Can you work these out from the model? Positions are in its coordinate system, mm. A direction names the side the tool comes from. Coordinates: 2 decimals unless noted, no trailing zeros. Order: outer loops, then holes, each group sorted by start corner. A loop starts at its lowest first (then second) coordinate and runs counter-clockwise, first axis right, second up. Notation, with made-up numbers: (76, -14) -> (133, -14) arc R16 ccw to (133, 3) -> close; hole circle Ø1 at (64, 48). An arc over 180 degrees is marked (long way). Answer in a Markdown table with one row per item.
```python
from build123d import *

# Parameters (mm, degrees)
SKETCH_2_W          = 37
SKETCH_2_H          = 13
EXTRUDE_2_DEPTH     = 3
SKETCH_3_R          = 1.5
CUT_EXTRUDE_2_DEPTH = 3
SKETCH_4_W          = 37
SKETCH_4_H          = 4
EXTRUDE_3_DEPTH     = 15
FILLET_4_R          = 3
FILLET_5_R          = 3
SKETCH_5_R          = 1.5
CUT_EXTRUDE_3_DEPTH = 10
FILLET_6_R          = 3


with BuildPart() as part:
    # 草图2 → 凸台-拉伸2 (new body)
    with BuildSketch(Plane(origin=(0, 0, 0), x_dir=(1, 0, 0), z_dir=(0, 1, 0))):
        Rectangle(SKETCH_2_W, SKETCH_2_H)
    extrude(amount=EXTRUDE_2_DEPTH)

    # 草图3 → 切除-拉伸2 (cut)
    with BuildSketch(Plane.XZ):
        with Locations(Location((-14.5, 0, 0), (0, 0, 270))):
            Circle(SKETCH_3_R)
        with Locations(Location((14.5, 0, 0), (0, 0, 270))):
            Circle(SKETCH_3_R)
    extrude(amount=-CUT_EXTRUDE_2_DEPTH, mode=Mode.SUBTRACT)

    # 草图4 → 凸台-拉伸3 (add)
    with BuildSketch(Plane.XZ):
        with Locations((0, -8.5)):
            Rectangle(SKETCH_4_W, SKETCH_4_H)
    extrude(amount=-EXTRUDE_3_DEPTH)

    # 圆角4
    fillet_4_edges = [part.edges().sort_by_distance(p)[0] for p in [
        (18.5, 15, -8.5),
    ]]
    fillet(fillet_4_edges, radius=FILLET_4_R)

    # 圆角5
    fillet_5_edges = [part.edges().sort_by_distance(p)[0] for p in [
        (-18.5, 15, -8.5),
    ]]
    fillet(fillet_5_edges, radius=FILLET_5_R)

    # 草图5 → 切除-拉伸3 (cut)
    with BuildSketch(Plane.XY.offset(-6.5)):
        with Locations((10, 9.01536156)):
            Circle(SKETCH_5_R)
        with Locations(Location((-10, 9.01536156, 0), (0, 0, 180))):
            Circle(SKETCH_5_R)
    extrude(amount=-CUT_EXTRUDE_3_DEPTH, mode=Mode.SUBTRACT)

    # 圆角6
    fillet_6_edges = [part.edges().sort_by_distance(p)[0] for p in [
        (-18.5, 1.5, 6.5),
        (18.5, 1.5, 6.5),
    ]]
    fillet(fillet_6_edges, radius=FILLET_6_R)


solid = part.part
```
(1) Suppose I cut it at A-A (x = 10). Please give me the cut outline in (y, z), and give its area (3 significant figures).
Response values:
| item | result |
|---|---|
| outline | (0, -10.5) -> (7.52, -10.5) -> (7.52, -6.5) -> (3, -6.5) -> (3, 6.5) -> (0, 6.5) -> close; (10.52, -10.5) -> (15, -10.5) -> (15, -6.5) -> (10.52, -6.5) -> close |
| area | 87.0 mm2 |
(2) I need wall thicknesses on line 1 (X direction, y = 1, z = 0); line 2 (Z direction, x = 8, y = 12.75); line 3 (Y direction, x = -5.5, z = 5.75). Which ranges of each line are inside material? Lowest first, please. Write a range as [from, to].
Response values:
| item | result |
|---|---|
| line 1 | [-18.5, -16], [-13, 13], [16, 18.5] |
| line 2 | [-10.5, -6.5] |
| line 3 | [0, 3] |
(3) We'd pull the mould along Z, two halves only. Please class faces 1 (the flat face through (0, 9, -6.5)), 2 (the cylindrical face through (17.64, 14.1, -8.47)), 3 (the cylindrical face through (-14.05, 1.48, -1.43)): +Z half, -Z half, draft (parallel to the pull), parting line (faces both ways), or undercut.
Response values:
| item | result |
|---|---|
| face 1 | +Z half |
| face 2 | draft |
| face 3 | undercut |
(4) Suppose I cut it at D-D (x = -14.5). Please give me the cut outline in (y, z), and give its area (3 significant figures).
Response values:
| item | result |
|---|---|
| outline | (0, -10.5) -> (15, -10.5) -> (15, -6.5) -> (3, -6.5) -> (3, -1.5) -> (0, -1.5) -> close; (0, 1.5) -> (3, 1.5) -> (3, 6.5) -> (0, 6.5) -> close |
| area | 90.0 mm2 |
(5) Suppose I cut it at B-B (y = 2.25). Please give me the cut outline in (x, z), and give its area (3 significant figures).
Response values:
| item | result |
|---|---|
| outline | (-18.5, -10.5) -> (18.5, -10.5) -> (18.5, 3.5) arc R3 ccw to (15.5, 6.5) -> (-15.5, 6.5) arc R3 ccw to (-18.5, 3.5) -> close; hole circle Ø3 at (-14.5, 0); hole circle Ø3 at (14.5, 0) |
| area | 611 mm2 |
(6) On a 3-axis mill with a long thin cutter (end or side, diameter ignored), from which of +Z, -Z, +X, -X, +Y, -Y can I reach the whole of each face in a straight line? I mean faces 4 (the flat face through (-18.5, 5, -7)), 5 (the flat face through (0, 3, 0)). Say none if no direction works.
Response values:
| item | result |
|---|---|
| face 4 | +Z, -Z, -X, +Y, -Y |
| face 5 | +Z, +X, -X, +Y |
(7) Suppose I cut it at C-C (z = 0). Please give me the cut outline in (x, y).
Response values:
| item | result |
|---|---|
| outline | (-18.5, 0) -> (-16, 0) -> (-16, 3) -> (-18.5, 3) -> close; (-13, 0) -> (13, 0) -> (13, 3) -> (-13, 3) -> close; (16, 0) -> (18.5, 0) -> (18.5, 3) -> (16, 3) -> close |
(8) Will these pins go through, and if not, where does the flat tip stop? pin 1 Ø2.5 at (x, z) = (-14.5, 0) entering from +Y; pin 2 Ø4 at (x, y) = (-12, 9) entering from +Z; pin 3 Ø1 at (x, z) = (2, -2) entering from +Y.
Response values:
| item | result |
|---|---|
| pin 1 | through |
| pin 2 | z = -6.5 |
| pin 3 | y = 3 |
